Autodesk Inventor part; units mm, degrees
ref_plane "YZ Plane" through (0, 0, 0) normal (1, 0, 0) x (0, 1, 0)
ref_plane "XZ Plane" through (0, 0, 0) normal (0, 1, 0) x (-1, 0, 0)
ref_plane "XY Plane" through (0, 0, 0) normal (0, 0, 1) x (1, 0, 0)
sketch "草圖1" plane through (0, 0, 0) normal (0, 1, 0) x (-1, 0, 0)
  line L0 (0, 0) -> (-20, 0)
  line L1 (-20, 0) -> (-20, -20)
  line L2 (-20, -20) -> (0, -20)
  line L3 (0, -20) -> (0, 0)
  line L4 (-20, 0) -> (-30, 0)
  line L5 (-30, 0) -> (-30, -30)
  line L6 (-30, -30) -> (-20, -30)
  line L7 (-20, -30) -> (-20, 0)
  line L8 (-30, -30) -> (-50, -30)
  line L9 (-50, -30) -> (-50, 10)
  line L10 (-50, 10) -> (-30, 10)
  line L11 (-30, 10) -> (-30, -30)
  dimension "d0" = 20
  dimension "d1" = 20
  dimension "d2" = 20
  dimension "d3" = 10
  dimension "d4" = 30
  dimension "d5" = 40
extrude "擠出1" add sketch "草圖1" along normal blind 10
fillet "圓角1" radius 20 2 edges at (50, 5, 10) (50, 5, -30)
fillet "圓角2" radius 10 2 edges at (0, 5, -20) (0, 5, 0)
sketch "草圖2" plane through (20, 0, -30) normal (-1, 0, 0) x (0, 0, 1)
  line L0 (10, 0) -> (10, 10)
  line L1 (10, 10) -> (-10, 30)
  line L2 (-10, 30) -> (-10, 0)
  line L3 (-10, 0) -> (10, 0)
  point P0 (30, 0)
  dimension "d10" = 20
  dimension "d11" = 30
extrude "擠出2" add sketch "草圖2" along normal blind 10
properties part number "44"
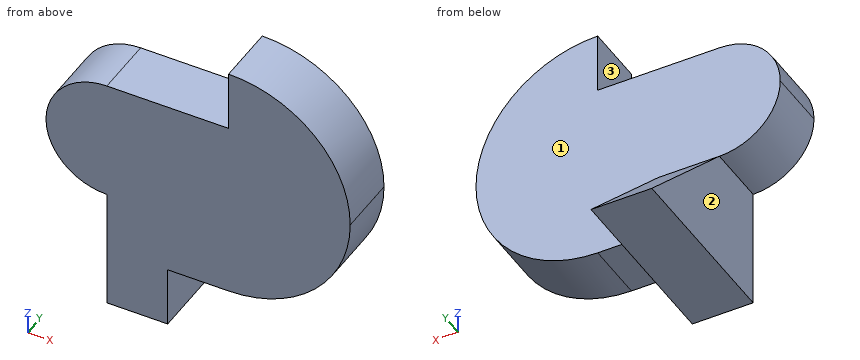
The model under review builds one solid part; all positions refer to its coordinate system, in mm. Face numbers are marked on the shaded views. A direction names the side the tool comes from. Give positions to 0.01 mm unless a question says otherwise; leave off trailing zeros. Write each loop counter-clockwise with the first axis right and the second up, starting at its lowest first coordinate (ties: lowest second). Pieces come first, ordered by that corner, then holes. Notation, with made-up numbers: (-38, 26) -> (-9, 26) arc R19 cw to (-9, 47) -> close; hole circle Ø1 at (-8, 39.25). An arc over 180 degrees is marked (long way). Put each result on its own line as item: value.
(1) Tool access review of the marked faces 1, 2 and 3: name each direction out of +Z, -Z, +X, -X, +Y, -Y from which nothing blocks a thin tool from reaching the whole face with its end or side.
Results are:
face 1: +Z, +X, +Y
face 2: -Z, -X, +Y, -Y
face 3: +Z, -X, +Y, -Y
(2) To check wall thickness, follow probe 1 along Y at (x, z) = (35.5, -26); probe 2 along Y at (x, z) = (11, -30); probe 3 along Z at (x, y) = (14, 28). State the ranges of each line that lie inside material, in increasing order. Write a range as from..to.
Results are:
probe 1: 0..10
probe 2: 0..20
probe 3: -40..-38
(3) For pin 1 Ø10 at (x, z) = (45, -12.5) entering from -Y; pin 2 Ø11 at (y, z) = (7.5, 6) entering from -X; pin 3 Ø12 at (x, z) = (32, -16) entering from +Y; pin 4 Ø3 at (x, y) = (23.5, 5.5) entering from -Z, all flat-tipped, find the tip position at first contact; note any pin that passes through.
Results are:
pin 1: y = 0
pin 2: x = 30
pin 3: y = 10
pin 4: z = -30
(4) We need section D-D, the plane y = 13.5. Give the boundary of the cut face in (x, z).
Results are:
outline: (10, -40) -> (20, -40) -> (20, -23.5) -> (10, -23.5) -> close
(5) We need section C-C, the plane z = -36. Give the boundary of the cut face in (x, y), and give its area (3 significant figures).
Results are:
outline: (10, 0) -> (20, 0) -> (20, 26) -> (10, 26) -> close
area: 260 mm²
(6) We need section B-B, the plane x = 16.5. Give the boundary of the cut face in (y, z).
Results are:
outline: (0, -40) -> (30, -40) -> (10, -20) -> (10, 0) -> (0, 0) -> close
